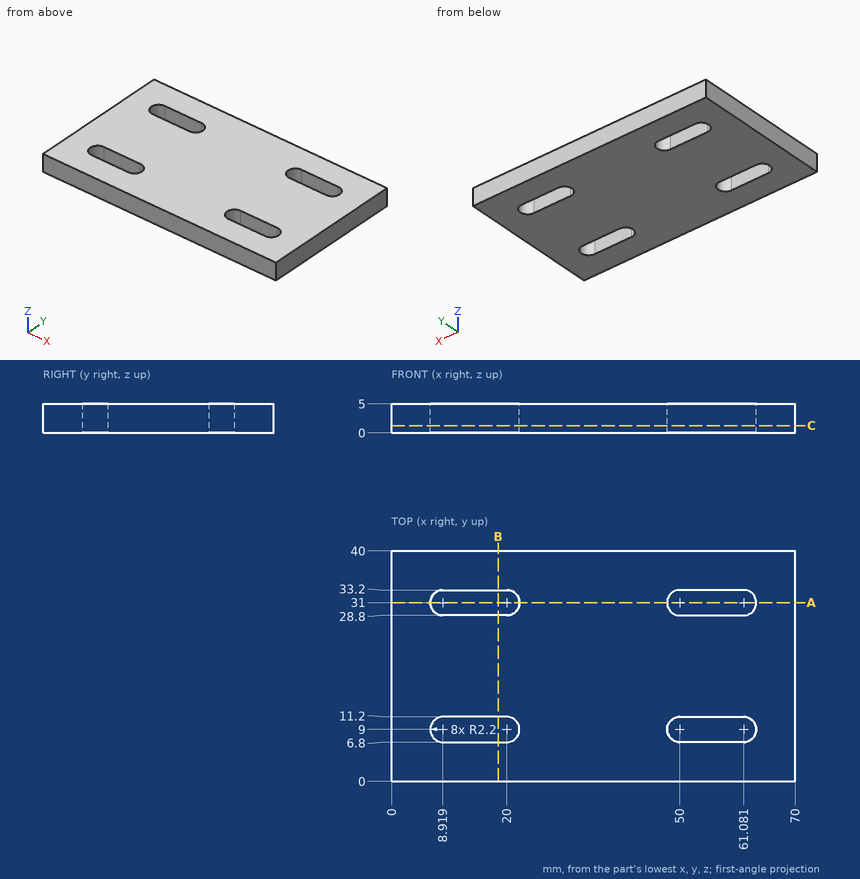
Source: three-view drawing plus pictorial views. Frame: mm from the lowest corner of the part. Coordinates: 2 decimals unless noted, no trailing zeros. Order: outer loops, then holes, each group sorted by start corner. A loop starts at its lowest first (then second) coordinate and runs counter-clockwise, first axis right, second up. Notation, with made-up numbers: M -12.75,14.25 L 8.25,14.25 A22 ccw 8.25,51.25 Z; hole C -38.5,12.25 d6. An arc over 180 degrees is marked long. One line per question, with ' | ' between items.
Item 1: Section A-A (y = 31). Output: boundary loops of the cut face in (x, z), then the cut area to 3 significant figures.
Geometry results:
outline: M 0,0 L 6.72,0 L 6.72,5 L 0,5 Z; M 22.2,0 L 47.8,0 L 47.8,5 L 22.2,5 Z; M 63.28,0 L 70,0 L 70,5 L 63.28,5 Z | area: 195 mm^2
Item 2: Section C-C (z = 1.25). Output: boundary loops of the cut face in (x, y), then the cut area to 3 significant figures.
Geometry results:
outline: M 0,0 L 70,0 L 70,40 L 0,40 Z; hole M 8.92,6.8 L 20,6.8 A2.2 ccw 20,11.2 L 8.92,11.2 A2.2 ccw Z; hole M 8.92,28.8 L 20,28.8 A2.2 ccw 20,33.2 L 8.92,33.2 A2.2 ccw Z; hole M 50,6.8 L 61.08,6.8 A2.2 ccw 61.08,11.2 L 50,11.2 A2.2 ccw Z; hole M 50,28.8 L 61.08,28.8 A2.2 ccw 61.08,33.2 L 50,33.2 A2.2 ccw Z | area: 2,540 mm^2
Item 3: Section B-B (x = 18.5). Output: boundary loops of the cut face in (y, z), then the cut area to 3 significant figures.
Geometry results:
outline: M 0,0 L 6.8,0 L 6.8,5 L 0,5 Z; M 11.2,0 L 28.8,0 L 28.8,5 L 11.2,5 Z; M 33.2,0 L 40,0 L 40,5 L 33.2,5 Z | area: 156 mm^2
Item 4: Ray query, line 1 along X through (y, z) = (31, 3.95); line 2 along Y through (x, z) = (12.5, 0.7); line 3 along X through (y, z) = (10.5, 4.1). Return the intervals inside material, ascending.
Geometry results:
line 1: x = 0 to 6.72, 22.2 to 47.8, 63.28 to 70 | line 2: y = 0 to 6.8, 11.2 to 28.8, 33.2 to 40 | line 3: x = 0 to 7.31, 21.61 to 48.39, 62.69 to 70
